Autodesk Inventor part; units mm, degrees
ref_plane "YZ Plane" through (0, 0, 0) normal (1, 0, 0) x (0, 1, 0)
ref_plane "XZ Plane" through (0, 0, 0) normal (0, 1, 0) x (-1, 0, 0)
ref_plane "XY Plane" through (0, 0, 0) normal (0, 0, 1) x (1, 0, 0)
sketch "Sketch1" plane through (0, 0, 0) normal (0, 1, 0) x (-1, 0, 0)
  line L0 (-9.22, 34.5) -> (9.22, 34.5)
  line L1 (9.22, 34.5) -> (9.22, -34.5)
  line L2 (9.22, -34.5) -> (-9.22, -34.5)
  line L3 (-9.22, -34.5) -> (-9.22, 34.5)
  line L4 (-9.22, 34.5) -> (9.22, -34.5) construction
  line L5 (9.22, 34.5) -> (-9.22, -34.5) construction
  point P0 (0, 0)
  dimension "d0" = 18.44
  dimension "d1" = 69
extrude "Extrusion1" add sketch "Sketch1" along normal blind 5.5
sketch "Sketch4" plane through (0, 5.5, 0) normal (0, 1, 0) x (1, 0, 0)
  circle A0 centre (-1.16, 19.65) radius 2.4879
  line L0 (-9.22, 34.5) -> (-9.22, -34.5)
  line L1 (-9.22, -34.5) -> (9.22, -34.5)
  point P0 (0, 0)
  dimension "d6" = 8.06
  dimension "d7" = 54.15
hole "Hole1" at (-1.16, 5.5, -19.65) direction (0, -1, 0) diameter 3.5 depth 10.5 tip angle 118 counterbore diameter 6 counterbore depth 2.3
sketch "Sketch5" plane through (0, 5.5, 0) normal (0, 1, 0) x (1, 0, 0)
  circle A0 centre (-1.16, -20.15) radius 2.6607
  line L0 (-9.22, 34.5) -> (-9.22, -34.5)
  line L1 (-9.22, -34.5) -> (9.22, -34.5)
  point P0 (0, 0)
  dimension "d15" = 8.06
  dimension "d16" = 14.35
hole "Hole2" at (-1.16, 5.5, 20.15) direction (0, -1, 0) diameter 3.5 depth 10.5 tip angle 118 counterbore diameter 6 counterbore depth 2.3
sketch "Sketch6" plane through (0, 5.5, 0) normal (0, 1, 0) x (1, 0, 0)
  line L0 (-9.22, -34.5) -> (9.22, -34.5)
  line L1 (-9.22, 34.5) -> (-9.22, -34.5)
  line L2 (6.22, -34.5) -> (-9.22, -34.5)
  line L3 (-9.22, -34.5) -> (-9.22, 34.5)
  line L4 (-9.22, 34.5) -> (6.22, 34.5)
  line L5 (6.22, 34.5) -> (6.22, -34.5)
  line L6 (9.22, -34.5) -> (9.22, 34.5)
  line L7 (6.22, -15.65) -> (-6.2399, -15.65)
  line L8 (-6.2399, -15.65) -> (-6.2399, -24.65)
  line L9 (-6.2399, -24.65) -> (6.22, -24.65)
  line L10 (6.22, 15.15) -> (-6.2399, 15.15)
  line L11 (-6.2399, 15.15) -> (-6.2399, 24.15)
  line L12 (-6.2399, 24.15) -> (6.22, 24.15)
  circle A0 centre (-1.16, -20.15) radius 3
  circle A1 centre (-1.16, 19.65) radius 3
  point P0 (0, 0)
  dimension "d24" = 3
  dimension "d25" = 9
  dimension "d26" = 9
  dimension "d27" = 4.5
  dimension "d28" = 4.5
extrude "Extrusion2" cut sketch "Sketch6" against normal blind 9 contours L1 L4 L5 L12 L11 L10 L7 L8 L9 L0
properties part number "support_2"
Check sheet for the modelled part. Datum: model origin and axes. Units: mm. A direction names the side the tool comes from. Give positions to 0.01 mm unless a question says otherwise; leave off trailing zeros. Loops run counter-clockwise (first coordinate to the right, second up) from the corner with the lowest first, then second, coordinate; pieces in that order, holes last. Notation, with made-up numbers: M -38.5,54.25 L -14.5,54.25 A24 ccw -14.5,67.25 Z; hole C -12,46.5 d3. An arc over 180 degrees is marked long. Answer as CSV lines item,"result".
Item 1: Scan lines: L1, parallel to Z at x = -1.16, y = 5.05; L2, parallel to X at y = 1.2, z = 20.15; L3, parallel to Z at x = -1.16, y = 2.4. Record each from-to range of solid material in increasing order.
Reply:
L1,"-24.15 to -22.65, -16.65 to -15.15, 15.65 to 17.15, 23.15 to 24.65"
L2,"-6.24 to -2.91, 0.59 to 9.22"
L3,"-24.15 to -21.4, -17.9 to -15.15, 15.65 to 18.4, 21.9 to 24.65"
Item 2: Sectioned sample at D-D, the plane y = 1.55. Enter the section's corners in (x, z).
Reply:
outline,"M -6.24,-24.15 L 6.22,-24.15 L 6.22,-34.5 L 9.22,-34.5 L 9.22,34.5 L 6.22,34.5 L 6.22,24.65 L -6.24,24.65 L -6.24,15.65 L 6.22,15.65 L 6.22,-15.15 L -6.24,-15.15 Z; hole C -1.16,-19.65 d3.5; hole C -1.16,20.15 d3.5"
Item 3: Depth check by flat-ended pin: pin 1 Ø4.5 at (x, z) = (-1.16, 20.15) entering from +Y; pin 2 Ø2 at (x, y) = (3, 4.5) entering from +Z. Enter the tip coordinate at first touch or a pass-through.
Reply:
pin 1,"y = 3.2"
pin 2,"z = 24.65"
Item 4: Sectioned sample at B-B, the plane y = 4.6. Enter the section's corners in (x, z).
Reply:
outline,"M -6.24,-24.15 L 6.22,-24.15 L 6.22,-34.5 L 9.22,-34.5 L 9.22,34.5 L 6.22,34.5 L 6.22,24.65 L -6.24,24.65 L -6.24,15.65 L 6.22,15.65 L 6.22,-15.15 L -6.24,-15.15 Z; hole C -1.16,-19.65 d6; hole C -1.16,20.15 d6"
Item 5: Sectioned sample at A-A, the plane x = -1.16. Enter the section's corners in (y, z).
Reply:
outline,"M 0,-24.15 L 5.5,-24.15 L 5.5,-22.65 L 3.2,-22.65 L 3.2,-21.4 L 0,-21.4 Z; M 0,-17.9 L 3.2,-17.9 L 3.2,-16.65 L 5.5,-16.65 L 5.5,-15.15 L 0,-15.15 Z; M 0,15.65 L 5.5,15.65 L 5.5,17.15 L 3.2,17.15 L 3.2,18.4 L 0,18.4 Z; M 0,21.9 L 3.2,21.9 L 3.2,23.15 L 5.5,23.15 L 5.5,24.65 L 0,24.65 Z"
Item 6: Draft check along Z on faces 6 (the face through (-6.24, 3, 20)), 7 (the face through (8, 3, -34.5)), 8 (the face through (-0.01, 4.33, 22.92)). Enter one of: pulls with the +Z half, pulls with the -Z half, needs draft (parallel to the pull), parting line crosses it, or undercut.
Reply:
face 6,"needs draft"
face 7,"pulls with the -Z half"
face 8,"undercut"
Item 7: Sectioned sample at C-C, the plane z = 20.15. Enter the section's corners in (x, y), then the cut area to 3 significant figures.
Reply:
outline,"M -6.24,0 L -2.91,0 L -2.91,3.2 L -4.16,3.2 L -4.16,5.5 L -6.24,5.5 Z; M 0.59,0 L 9.22,0 L 9.22,5.5 L 1.84,5.5 L 1.84,3.2 L 0.59,3.2 Z"
area,"60.0 mm^2"
Item 8: Set-up check for faces 1 (the face through (0, 3, -24.15)), 2 (the face through (0, 3, 24.65)), 3 (the face through (8, 3, 34.5)), 4 (the face through (0, 3.2, -18)), 5 (the face through (6.22, 3, 0)): record each of +Z, -Z, +X, -X, +Y, -Y from which the full face is reachable in a straight line by a thin tool's end or side.
Reply:
face 1,"-Z, -X, +Y, -Y"
face 2,"+Z, -X, +Y, -Y"
face 3,"+Z, +X, -X, +Y, -Y"
face 4,"+Y"
face 5,"-X, +Y, -Y"
